Geometry: see drawing. Coordinates: mm, zero at the bounding-box minimum. Give positions to 0.01 mm unless a question says otherwise; leave off trailing zeros. Loops run counter-clockwise (first coordinate to the right, second up) from the corner with the lowest first, then second, coordinate; pieces in that order, holes last. Notation, with made-up numbers: (-10.75, 24.25) -> (-0.75, 24.25) arc R12 cw to (-0.75, 47.25) -> close; hole circle Ø9 at (71, -17). An arc over 180 degrees is marked (long way). Return JSON: item names as keys, results as strings. Group by question number.
(1) Cut plane B-B on y = 6.75. Return loops of the section in (x, z), then the cut area to 3 significant figures.
(2) Draft query along X for the marked faces 1, 2, 3 and 4. Return one class per face: released by +X, released by -X, zero draft, split by the parting line, or undercut.
(3) Ray query, line 1 (Z direction, x = 0.5, y = 6.75); line 2 (X direction, y = 8.25, z = 25); line 3 (Y direction, x = 33.5, z = 34). Return the intervals inside material, ascending. Write a range as from..to.
(4) Pin query (flat end, axial travel): pin 1 (7 mm diameter, centred on x = 19.3, z = 35, fed in from +Y); pin 2 (8 mm diameter, centred on x = 12.5, y = 5, fed in from +Z); pin 3 (3 mm diameter, centred on x = 15, y = 4, fed in from -Z). Return the tip coordinate at first contact, or that it passes through.
(5) Cut plane C-C on x = 19.3. Return loops of the section in (y, z), then the cut area to 3 significant figures.
(6) Cut plane D-D on y = 12.5. Return loops of the section in (x, z).
(7) Cut plane A-A on z = 6. Return loops of the section in (x, y).
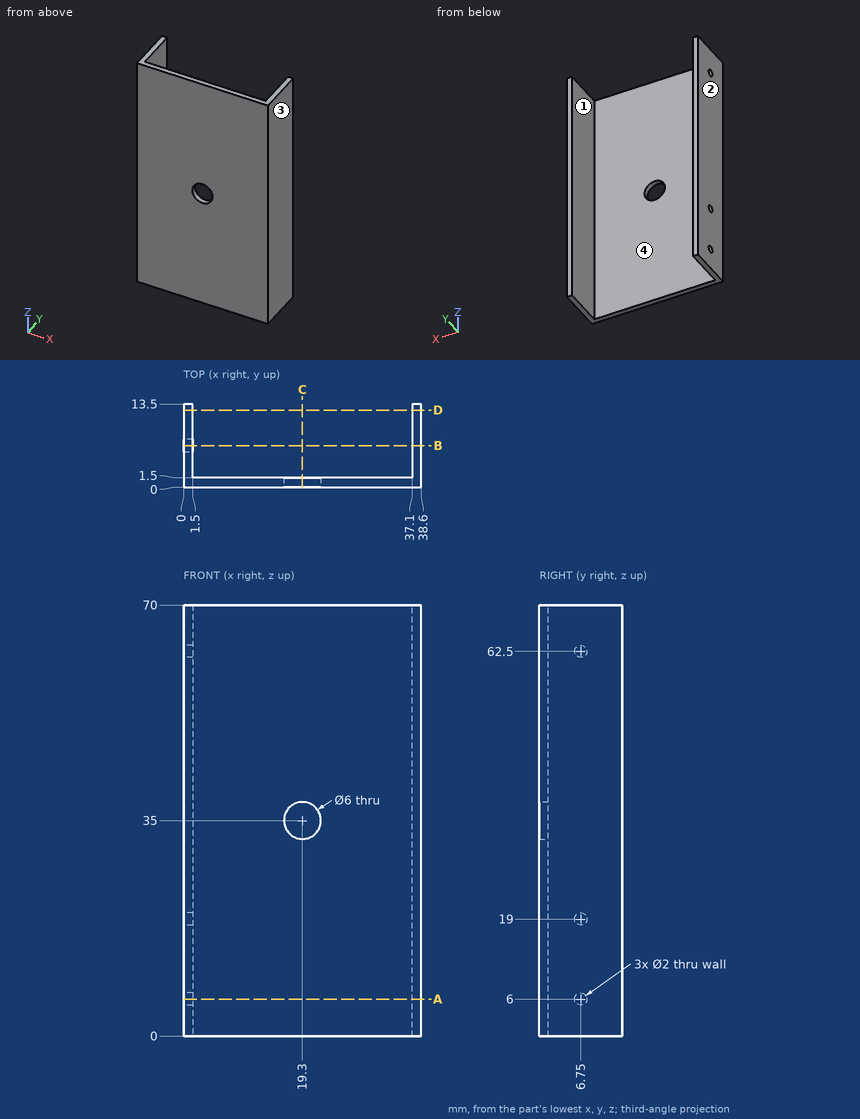
Answers:
{
 "1": {"outline": "(0, 0) -> (1.5, 0) -> (1.5, 5) -> (0, 5) -> close; (0, 7) -> (1.5, 7) -> (1.5, 18) -> (0, 18) -> close; (0, 20) -> (1.5, 20) -> (1.5, 61.5) -> (0, 61.5) -> close; (0, 63.5) -> (1.5, 63.5) -> (1.5, 70) -> (0, 70) -> close; (37.1, 0) -> (38.6, 0) -> (38.6, 70) -> (37.1, 70) -> close", "area": "201 mm²"},
 "2": {"face 1": "undercut", "face 2": "released by -X", "face 3": "released by +X", "face 4": "undercut"},
 "3": {"line 1": "0..5, 7..18, 20..61.5, 63.5..70", "line 2": "0..1.5, 37.1..38.6", "line 3": "0..1.5"},
 "4": {"pin 1": "y = 1.5", "pin 2": "z = 70", "pin 3": "through"},
 "5": {"outline": "(0, 0) -> (1.5, 0) -> (1.5, 32) -> (0, 32) -> close; (0, 38) -> (1.5, 38) -> (1.5, 70) -> (0, 70) -> close", "area": "96.0 mm²"},
 "6": {"outline": "(0, 0) -> (1.5, 0) -> (1.5, 70) -> (0, 70) -> close; (37.1, 0) -> (38.6, 0) -> (38.6, 70) -> (37.1, 70) -> close"},
 "7": {"outline": "(0, 0) -> (38.6, 0) -> (38.6, 13.5) -> (37.1, 13.5) -> (37.1, 1.5) -> (1.5, 1.5) -> (1.5, 5.75) -> (0, 5.75) -> close; (0, 7.75) -> (1.5, 7.75) -> (1.5, 13.5) -> (0, 13.5) -> close"}
}
